```python
from build123d import *

# Parameters (mm, degrees)
F0_R      = 17.9
F1_DEPTH  = 50
F2_R      = 5.1
F3_DEPTH  = 3
F4_R      = 1.585
F5_DEPTH  = 1
F6_R      = 6.5
F7_DEPTH  = 4.5
F8_DEPTH  = 71
F9_W      = 6
F9_H      = 2.8
F10_DEPTH = 1
F11_W     = 3.8
F11_H     = 0.5
F12_DEPTH = 6
F13_SIZE  = 0.8
F14_R     = 0.5
F15_SIZE  = 0.3
F17_DEPTH = 1
F19_SIZE  = 0.5
F20_SIZE  = 0.5
F21_R     = 1.5
F22_R     = 0.8
F23_R     = 1.5
F24_DEPTH = 2
F25_COUNT = 3
F25_ANGLE = 180


with BuildPart() as f1:
    # F0 (on Top) → F1 (new body)
    with BuildSketch(Plane.XY):
        Circle(F0_R)
    extrude(amount=F1_DEPTH)

    # F2 (on face) → F3 (join)
    with BuildSketch(Plane(origin=(0, 0, 0), x_dir=(1, 0, 0), z_dir=(0, 0, -1))):
        Circle(F2_R)
    extrude(amount=F3_DEPTH)

    # F4 (on face) → F5 (join)
    with BuildSketch(Plane(origin=(0, 0, -3), x_dir=(1, 0, 0), z_dir=(0, 0, -1))):
        Circle(F4_R)
    extrude(amount=F5_DEPTH)

    # F6 (on face) → F7 (join)
    with BuildSketch(Plane.XY.offset(50)):
        Circle(F6_R)
    extrude(amount=F7_DEPTH)

    # F8 (add): a face of the model
    f8_faces = [f1.faces().sort_by_distance(p)[0] for p in [
        (0, 0, -4),
    ]]
    extrude(f8_faces, amount=-F8_DEPTH)



with BuildPart() as f10:
    # F9 (on face) → F10 (new body)
    with BuildSketch(Plane(origin=(0, 0, 0), x_dir=(1, 0, 0), z_dir=(0, 0, -1))):
        with Locations((0, -14.2)):
            Rectangle(F9_W, F9_H)
    extrude(amount=F10_DEPTH)

    # F11 (on face) → F12 (join)
    with BuildSketch(Plane(origin=(0, 0, -1), x_dir=(1, 0, 0), z_dir=(0, 0, -1))):
        with Locations((0, -13.95)):
            Rectangle(F11_W, F11_H)
    extrude(amount=F12_DEPTH)

    # F13
    f13_edges = [f10.edges().sort_by_distance(p)[0] for p in [
        (1.9, 13.95, -7),
        (-1.9, 13.95, -7),
    ]]
    chamfer(f13_edges, length=F13_SIZE)

    # F14
    f14_edges = [f10.edges().sort_by_distance(p)[0] for p in [
        (3, 15.6, -0.5),
        (-3, 15.6, -0.5),
        (3, 12.8, -0.5),
        (-3, 12.8, -0.5),
    ]]
    fillet(f14_edges, radius=F14_R)

    # F15
    f15_edges = [f10.edges().sort_by_distance(p)[0] for p in [
        (0, 12.8, -1),
    ]]
    chamfer(f15_edges, length=F15_SIZE)

    # F16 (on face) → F17 (cut)
    with BuildSketch(Plane(origin=(0, 14.2, 0), x_dir=(-1, 0, 0), z_dir=(0, 1, 0))):
        with BuildLine():
            Line((0.9, -4.6), (0.9, -3.9))
            ThreePointArc((0.9, -3.9), (0, -3), (-0.9, -3.9))
            Line((-0.9, -3.9), (-0.9, -4.6))
            ThreePointArc((-0.9, -4.6), (0, -5.5), (0.9, -4.6))
        make_face()
    extrude(amount=-F17_DEPTH, mode=Mode.SUBTRACT)


with BuildPart() as f1_1:
    add(f1.part)

    add(f10.part)  # F18 merges F10
    # F18: F10 across plane
    add(f10.part.mirror(Plane.XZ))

    # F19
    f19_edges = [f1_1.edges().sort_by_distance(p)[0] for p in [
        (-5.1, 0, -3),
    ]]
    chamfer(f19_edges, length=F19_SIZE)

    # F20
    f20_edges = [f1_1.edges().sort_by_distance(p)[0] for p in [
        (-6.5, 0, 54.5),
    ]]
    chamfer(f20_edges, length=F20_SIZE)

    # F21
    f21_edges = [f1_1.edges().sort_by_distance(p)[0] for p in [
        (-17.9, 0, 50),
    ]]
    fillet(f21_edges, radius=F21_R)

    # F22
    f22_edges = [f1_1.edges().sort_by_distance(p)[0] for p in [
        (-1.585, 0, 67),
    ]]
    fillet(f22_edges, radius=F22_R)

    # F25: F24 ×3 about axis
    f25_axis = Axis((0, 0, 0), (0, 0, 1))


with BuildPart() as f24:
    # F23 (on face) → F24 (new body)
    with BuildSketch(Plane.XY.offset(50)):
        with Locations((0.654199453, -12.4828691844)):
            Circle(F23_R)
    extrude(amount=-F24_DEPTH)


with BuildPart() as f1_2:
    add(f1_1.part)
    for i in range(1, F25_COUNT):
        add(f24.part.rotate(f25_axis, i * F25_ANGLE / (F25_COUNT - 1)), mode=Mode.SUBTRACT)

    # F25#seed: cut F24
    add(f24.part, mode=Mode.SUBTRACT)


solid = f1_2.part
```
CAD build for the part. Positions are in the model's coordinates, mm. A direction names the side the tool comes from. Round coordinates to 2 decimals unless told otherwise and drop trailing zeros. Order: outer loops, then holes, each group sorted by start corner. A loop starts at its lowest first (then second) coordinate and runs counter-clockwise, first axis right, second up.
Q1. Slice it at B-B (x = 0). State how many separate pieces and enclosed holes the cut face has, and give its area (3 significant figures).
Q2. Slice it at A-A (z = 2). Write the cut outline in (x, y).
Q3. Wall check: L1, parallel to Z at x = -10, y = -10; L2, parallel to Z at x = 4.5, y = 2.5; L3, parallel to X at y = 4, z = 11.5. Give the ranges that are in metal, low to high.
Q4. Drop flat-ended pins along their axis: pin 1 (6 mm diameter, centred on x = -2.5, z = 21.5, fed in from +Y); pin 2 (1 mm diameter, centred on x = -11.5, y = 10, fed in from +Z); pin 3 (1 mm diameter, centred on x = 13, y = 9, fed in from -Z). Give the stop position or say it passes through.
Q5. Two-plate mould, pull along X, no slides. Class faces 5 (the cylindrical face through (10.996, 0.459, 49.014)), 6 (the flat face through (-1, -14.2, -3)), 7 (the cylindrical face through (-1.26, 0.96, 60.27)), 8 (the cylindrical face through (0.459, -10.996, 49.014)): pulls with the +X half, pulls with the -X half, needs draft (parallel to the pull), parting line crosses it, or undercut.
Q6. Which spindle directions (+Z, -Z, +X, -X, +Y, -Y) get a long thin tool onto all of the face, cutting with end or side? Do faces 1 (the cylindrical face through (-1.26, 0.96, -3.49)), 2 (the cylindrical face through (-5.158, -3.955, 51.972)), 3 (the flat face through (0, 0, 67)), 4 (the flat face through (-1, 13.7, -3)). Say none if no direction does.
Results below:
1. separate pieces: 3
1. enclosed holes: 0
1. area: 1,920 mm2
2. outline: circle Ø35.8 at (0, 0)
3. L1: z = 0 to 50
3. L2: z = 0 to 54.5
3. L3: x = -17.45 to 17.45
4. pin 1: stops at y = 17.9
4. pin 2: stops at z = 50
4. pin 3: stops at z = 0
5. face 5: undercut
5. face 6: needs draft
5. face 7: parting line crosses it
5. face 8: undercut
6. face 1: -Z
6. face 2: +Z
6. face 3: +Z, +X, -X, +Y, -Y
6. face 4: -Z, +X, -X
